```python
from build123d import *

# Parameters (mm, degrees)
F0_W     = 40
F0_H     = 135
F1_DEPTH = 30
F2_W     = 80
F2_H     = 60
F3_DEPTH = 60
F4_W     = 80
F4_H     = 60
F4_R     = 27.5
F5_DEPTH = 25
F6_W     = 50.039211
F6_H     = 42.056428
F6_R     = 6
F7_DEPTH = 12


with BuildPart() as f1:
    # F0 (on Top) → F1 (new body)
    with BuildSketch(Plane.XY):
        Rectangle(F0_W, F0_H)
    extrude(amount=F1_DEPTH)

    # F2 (on Top) → F3 (join)
    with BuildSketch(Plane.XY):
        with Locations((10, 0)):
            Rectangle(F2_W, F2_H)
    extrude(amount=F3_DEPTH)

    # F4 (on face) → F5 (cut)
    with BuildSketch(Plane.XY.offset(60)):
        with Locations((10, 0)):
            Rectangle(F4_W, F4_H)
        Circle(F4_R, mode=Mode.SUBTRACT)
    extrude(amount=-F5_DEPTH, mode=Mode.SUBTRACT)

    # F6 (on face) → F7 (cut)
    with BuildSketch(Plane.XY.offset(30)):
        with Locations((-0.737083, 51.028214)):
            Rectangle(F6_W, F6_H)
        with Locations((0, 51.5)):
            Circle(F6_R, mode=Mode.SUBTRACT)
        with Locations((-0.737083, -51.028214)):
            Rectangle(F6_W, F6_H)
        with Locations((0, -51.5)):
            Circle(F6_R, mode=Mode.SUBTRACT)
    extrude(amount=-F7_DEPTH, mode=Mode.SUBTRACT)


solid = f1.part
```
CAD build for the part. Positions are in the model's coordinates, mm. A direction names the side the tool comes from. Give positions to 0.01 mm unless a question says otherwise; leave off trailing zeros. Loops run counter-clockwise (first coordinate to the right, second up) from the corner with the lowest first, then second, coordinate; pieces in that order, holes last. Notation, with made-up numbers: (77, 12) - (130, 12) arc R22 ccw to (130, 19) - close; hole circle Ø2 at (1, 46). An arc over 180 degrees is marked (long way). Put each result on its own line as item: value.
Q1. Probe line 1 along Z through (x, y) = (20.5, -29); line 2 along Z through (x, y) = (-5.5, -44.5); line 3 along X through (y, z) = (-59, 17). List the from-to ranges inside material, lowest first.
Filled in:
line 1: z = 0 to 35
line 2: z = 0 to 18
line 3: x = -20 to 20
Q2. Slice it at C-C (y = -51.5). Give the cut face in (x, z).
Filled in:
outline: (-20, 0) - (20, 0) - (20, 18) - (6, 18) - (6, 30) - (-6, 30) - (-6, 18) - (-20, 18) - close
Q3. Slice it at B-B (z = 8). Give the cut face in (x, y), plus the area to 3 significant figures.
Filled in:
outline: (-30, -30) - (-20, -30) - (-20, -67.5) - (20, -67.5) - (20, -30) - (50, -30) - (50, 30) - (20, 30) - (20, 67.5) - (-20, 67.5) - (-20, 30) - (-30, 30) - close
area: 7,800 mm²
Q4. Mould opens along Y. For faces 1 (the face through (9, 1, 0)), 2 (the face through (0, 45, 18)), 3 (the face through (-1.301, -57.357, 24.084)), 4 (the face through (0, -67.5, 9)) say: pulls with the +Y half, pulls with the -Y half, needs draft (parallel to the pull), parting line crosses it, or undercut.
Filled in:
face 1: needs draft
face 2: undercut
face 3: undercut
face 4: pulls with the -Y half
Q5. Flat gauge pins, fed straight in: pin 1 (14.5 mm diameter, centred on y = 42.5, z = 10, fed in from +X); pin 2 (9.5 mm diameter, centred on x = 1, y = 51.5, fed in from +Z); pin 3 (3 mm diameter, centred on y = 5, z = 44, fed in from -X). Where does each tip first touch, or does it go through?
Filled in:
pin 1: stops at x = 20
pin 2: stops at z = 30
pin 3: stops at x = -27.28
Q6. Slice it at D-D (x = 8). Give the cut face in (y, z), plus the area to 3 significant figures.
Filled in:
outline: (-67.5, 0) - (67.5, 0) - (67.5, 18) - (30, 18) - (30, 35) - (26.31, 35) - (26.31, 60) - (-26.31, 60) - (-26.31, 35) - (-30, 35) - (-30, 18) - (-67.5, 18) - close
area: 4,770 mm²
Q7. Tool access for faces 5 (the face through (-20, 48, 9)), 6 (the face through (0, 52, 30)), 7 (the face through (20, -49, 9)), 8 (the face through (27, 7, 35)), 9 (the face through (-20, -49, 9)): list every direction of +Z, -Z, +X, -X, +Y, -Y with a clear straight run to the whole face (end or side of a thin tool).
Filled in:
face 5: +Z, -Z, -X, +Y
face 6: +Z, +X, -X, +Y
face 7: +Z, -Z, +X, -Y
face 8: +Z
face 9: +Z, -Z, -X, -Y
Q8. Slice it at A-A (y = -24.5). Give the cut face in (x, z), plus the area to 3 significant figures.
Filled in:
outline: (-30, 0) - (50, 0) - (50, 35) - (12.49, 35) - (12.49, 60) - (-12.49, 60) - (-12.49, 35) - (-30, 35) - close
area: 3,420 mm²
